Geometry check sheet. Reference: drawing and pictorial views, mm from the part's lowest x, y, z. A direction names the side the tool comes from. Give positions to 0.01 mm unless a question says otherwise; leave off trailing zeros. Write each loop counter-clockwise with the first axis right and the second up, starting at its lowest first coordinate (ties: lowest second). Pieces come first, ordered by that corner, then holes. Notation, with made-up numbers: (82.5, 15.25) - (136.5, 15.25) arc R10 cw to (136.5, 27.25) - close; hole circle Ø7 at (-39.75, 16). An arc over 180 degrees is marked (long way). Put each result on its own line as item: value.
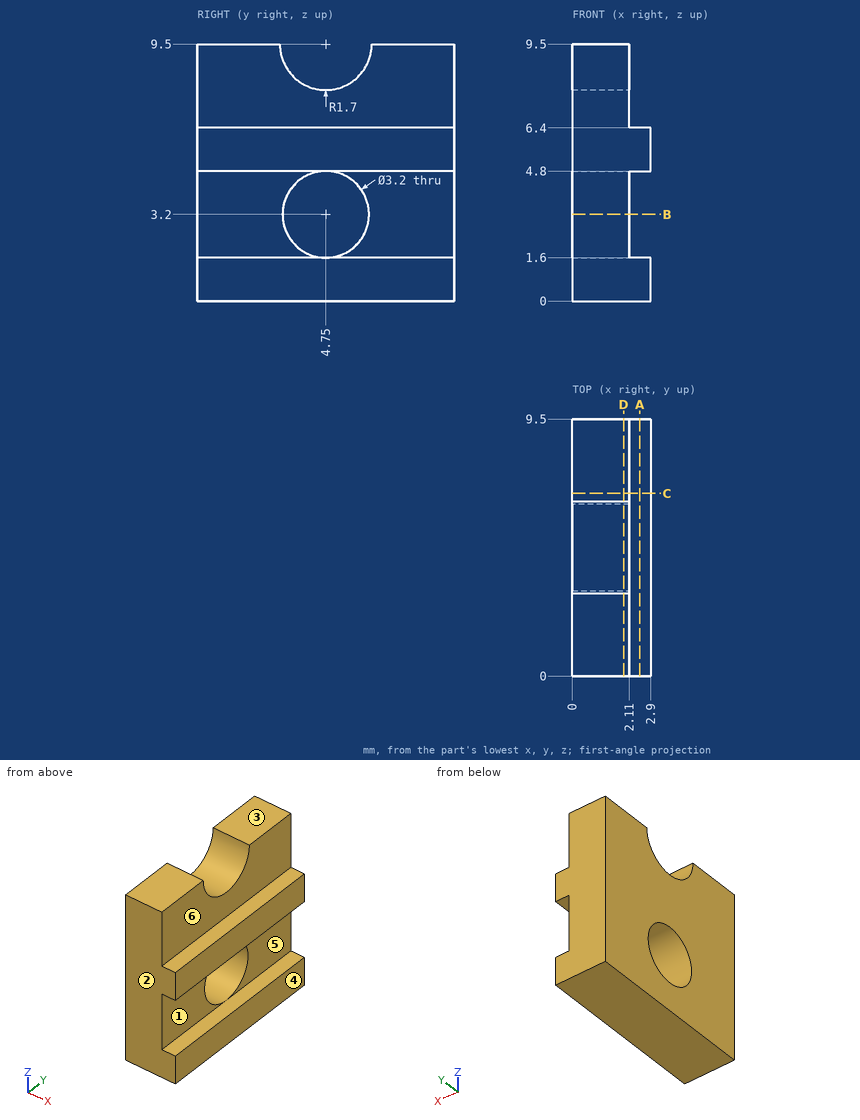
Q1. Section check D-D, the plane x = 1.9. Record the cut outline in (y, z), plus the area to 3 significant figures.
Answers follow:
outline: (0, 0) - (9.5, 0) - (9.5, 9.5) - (6.45, 9.5) arc R1.7 cw to (3.05, 9.5) - (0, 9.5) - close; hole circle Ø3.2 at (4.75, 3.2)
area: 77.7 mm2
Q2. Section check C-C, the plane y = 6.75. Record the cut outline in (x, z), plus the area to 3 significant figures.
Answers follow:
outline: (0, 0) - (2.9, 0) - (2.9, 1.6) - (2.11, 1.6) - (2.11, 4.8) - (2.9, 4.8) - (2.9, 6.4) - (2.11, 6.4) - (2.11, 9.5) - (0, 9.5) - close
area: 22.6 mm2
Q3. Go/stop test with a flat-tipped pin: pin 1 Ø2.5 at (y, z) = (6.5, 8.5) entering from +X. Record where the tip stops, or that it passes through.
Answers follow:
pin 1: stops at x = 2.11
Q4. Release check for a two-part mould opening along Z. For the marked faces 1, 2 and 3 record: released by +Z, released by -Z, zero draft, split by the parting line, or undercut.
Answers follow:
face 1: undercut
face 2: zero draft
face 3: released by +Z
Q5. Set-up check for the marked faces 4, 5 and 6: record each of +Z, -Z, +X, -X, +Y, -Y from which the full face is reachable in a straight line by a thin tool's end or side.
Answers follow:
face 4: +Z, -Z, +X, +Y, -Y
face 5: +X, +Y, -Y
face 6: +Z, +X, +Y, -Y
Q6. Section check A-A, the plane x = 2.5. Record the cut outline in (y, z), plus the area to 3 significant figures.
Answers follow:
outline: (0, 0) - (9.5, 0) - (9.5, 1.6) - (0, 1.6) - close; (0, 4.8) - (9.5, 4.8) - (9.5, 6.4) - (0, 6.4) - close
area: 30.4 mm2
Q7. Section check B-B, the plane z = 3.2. Record the cut outline in (x, y).
Answers follow:
outline: (0, 0) - (2.11, 0) - (2.11, 3.15) - (0, 3.15) - close; (0, 6.35) - (2.11, 6.35) - (2.11, 9.5) - (0, 9.5) - close
Q8. Scan lines: line 1 along Z through (x, y) = (1, 4.75); line 2 along Y through (x, z) = (0.55, 3.2); line 3 along Z through (x, y) = (2.2, 5.25). Record each from-to range of solid material in increasing order.
Answers follow:
line 1: z = 0 to 1.6, 4.8 to 7.8
line 2: y = 0 to 3.15, 6.35 to 9.5
line 3: z = 0 to 1.6, 4.8 to 6.4
